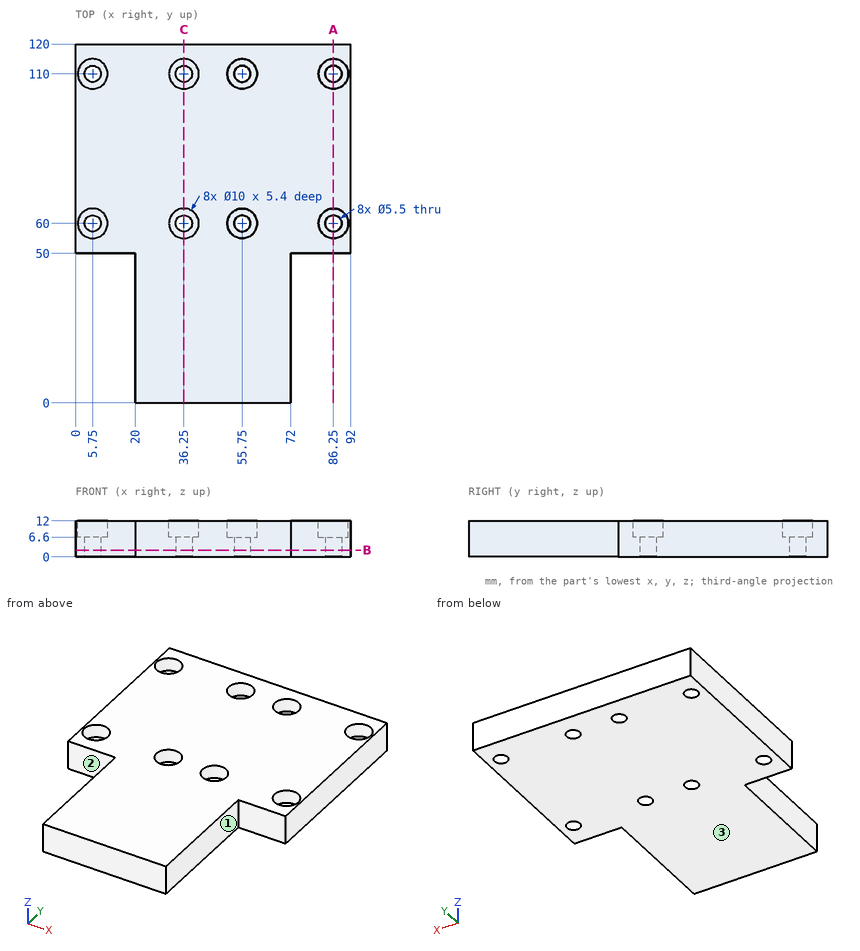
Verification items for this drawing (mm, ordinates from the low corner). A direction names the side the tool comes from. Round coordinates to 2 decimals unless told otherwise and drop trailing zeros. Write each loop counter-clockwise with the first axis right and the second up, starting at its lowest first coordinate (ties: lowest second). Pieces come first, ordered by that corner, then holes. Notation, with made-up numbers: M 45.5,5.5 L 80.5,5.5 A14 cw 80.5,21.5 Z; hole C -35,62 d11. An arc over 180 degrees is marked long. Write item = value, one per line. Start each with the question number.
1. Tool access check on the marked faces 1, 2 and 3. Record the directions out of +Z, -Z, +X, -X, +Y, -Y that give a thin tool (end or side, any length) a straight path to the whole face; none if there is none.
2. Section check C-C, the plane x = 36.25. Record the cut outline in (y, z), then the cut area to 3 significant figures.
3. Section check A-A, the plane x = 86.25. Record the cut outline in (y, z), then the cut area to 3 significant figures.
4. Section check B-B, the plane z = 2.25. State how many separate pieces and enclosed holes the cut face has, then the cut area to 3 significant figures.
5. Scan lines: line 1 (X direction, y = 110, z = 5); line 2 (Y direction, x = 86, z = 9.75); line 3 (Y direction, x = 86.25, z = 4). Record each from-to range of solid material in increasing order. Write a range as [from, to].
6. Gauge pin test, flat ends, axial feed: pin 1 (3 mm diameter, centred on y = 89, z = 7.5, fed in from -X); pin 2 (5 mm diameter, centred on x = 34.5, y = 111.5, fed in from +Z); pin 3 (4.5 mm diameter, centred on x = 55.75, y = 60, fed in from -Z); pin 4 (1 mm diameter, centred on y = 19.5, z = 10, fed in from +X). Record the tip position at first contact, or that the pin passes through.
Results found:
q1.face_1 = +Z, -Z, +X, -Y
q1.face_2 = +Z, -Z, -X, -Y
q1.face_3 = -Z, +X, -X, +Y, -Y
q2.outline = M 0,0 L 57.25,0 L 57.25,6.6 L 55,6.6 L 55,12 L 0,12 Z; M 62.75,0 L 107.25,0 L 107.25,6.6 L 105,6.6 L 105,12 L 65,12 L 65,6.6 L 62.75,6.6 Z; M 112.75,0 L 120,0 L 120,12 L 115,12 L 115,6.6 L 112.75,6.6 Z
q2.area = 1,260 mm^2
q3.outline = M 50,0 L 57.25,0 L 57.25,6.6 L 55,6.6 L 55,12 L 50,12 Z; M 62.75,0 L 107.25,0 L 107.25,6.6 L 105,6.6 L 105,12 L 65,12 L 65,6.6 L 62.75,6.6 Z; M 112.75,0 L 120,0 L 120,12 L 115,12 L 115,6.6 L 112.75,6.6 Z
q3.area = 659 mm^2
q4.separate_pieces = 1
q4.enclosed_holes = 8
q4.area = 8,850 mm^2
q5.line_1 = [0, 3], [8.5, 33.5], [39, 53], [58.5, 83.5], [89, 92]
q5.line_2 = [50, 55.01], [64.99, 105.01], [114.99, 120]
q5.line_3 = [50, 57.25], [62.75, 107.25], [112.75, 120]
q6.pin_1 = 0
q6.pin_2 = 6.6
q6.pin_3 = through
q6.pin_4 = 72
